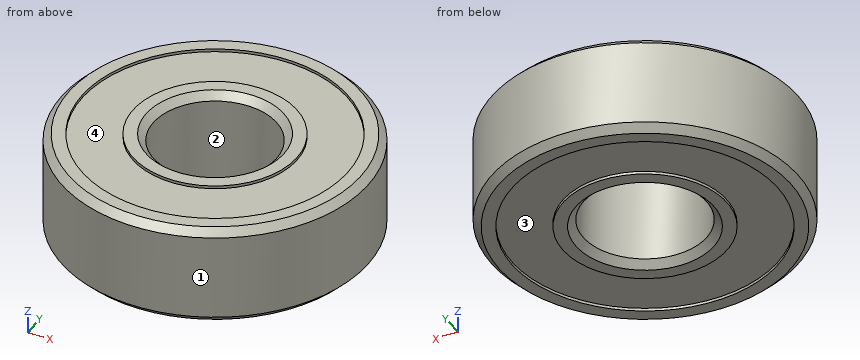
from build123d import *

# Parameters (mm, degrees)
ESQUISSE1_R        = 10.55
ESQUISSE1_R_2      = 9.15
BOSS_EXTRU_1_DEPTH = 3.45
ESQUISSE1_3_R      = 5.65
ESQUISSE1_3_R_2    = 4.25
BOSS_EXTRU_2_DEPTH = 3.45
ESQUISSE1_4_R      = 9.15
ESQUISSE1_4_R_2    = 5.65
BOSS_EXTRU_3_DEPTH = 3.25
CHANFREIN1_SIZE    = 0.5


with BuildPart() as part:
    # Esquisse1 → Boss.-Extru.1 (new body, symmetric)
    with BuildSketch(Plane.XY):
        Circle(ESQUISSE1_R)
        Circle(ESQUISSE1_R_2, mode=Mode.SUBTRACT)
    extrude(amount=BOSS_EXTRU_1_DEPTH, both=True)



with BuildPart() as body_2:
    # Esquisse1<3> → Boss.-Extru.2 (new body, symmetric)
    with BuildSketch(Plane.XY):
        Circle(ESQUISSE1_3_R)
        Circle(ESQUISSE1_3_R_2, mode=Mode.SUBTRACT)
    extrude(amount=BOSS_EXTRU_2_DEPTH, both=True)


with BuildPart() as part_1:
    add(part.part)

    add(body_2.part)  # Boss.-Extru.3 merges body 2
    # Esquisse1<4> → Boss.-Extru.3 (add, symmetric)
    with BuildSketch(Plane.XY):
        Circle(ESQUISSE1_4_R)
        Circle(ESQUISSE1_4_R_2, mode=Mode.SUBTRACT)
    extrude(amount=BOSS_EXTRU_3_DEPTH, both=True)

    # Chanfrein1
    chanfrein1_edges = [part_1.edges().sort_by_distance(p)[0] for p in [
        (-4.25, 0, -3.45),
        (-4.25, 0, 3.45),
        (-10.55, 0, -3.45),
        (-10.55, 0, 3.45),
    ]]
    chamfer(chanfrein1_edges, length=CHANFREIN1_SIZE)


solid = part_1.part
Verification items for the finished model (mm, model axes). Face numbers are marked on the shaded views. A direction names the side the tool comes from. Round coordinates to 2 decimals unless told otherwise and drop trailing zeros. Order: outer loops, then holes, each group sorted by start corner. A loop starts at its lowest first (then second) coordinate and runs counter-clockwise, first axis right, second up. Notation, with made-up numbers: (84, 82) -> (101, 82) arc R7 ccw to (101, 94) -> close; hole circle Ø8 at (11.25, -17.5). An arc over 180 degrees is marked (long way). Put each result on its own line as item: value.
1) Section check C-C (z = -1.5). Record the cut outline in (x, y), then the cut area to 3 significant figures.
Final values:
outline: circle Ø21.1 at (0, 0); hole circle Ø8.5 at (0, 0)
area: 293 mm^2
2) Mould release check, pull along X, two halves, no side actions. Record for the marked faces 1 and 2: +X half, -X half, draft (parallel to the pull), parting line (faces both ways), or undercut.
Final values:
face 1: parting line
face 2: undercut
3) Depth check by flat-ended pin: pin 1 (1.5 mm diameter, centred on y = 7, z = 1, fed in from -X); pin 2 (3 mm diameter, centred on x = 4.5, z = 0.5, fed in from +Y); pin 3 (1 mm diameter, centred on x = 8.5, z = 0.5, fed in from +Y). Enter the tip coordinate at first touch or a pass-through.
Final values:
pin 1: stops at x = -8.5
pin 2: stops at y = 10.11
pin 3: stops at y = 6.88
4) Set-up check for the marked faces 3 and 4: record each of +Z, -Z, +X, -X, +Y, -Y from which the full face is reachable in a straight line by a thin tool's end or side.
Final values:
face 3: -Z
face 4: +Z
5) Material ranges on line 1 (Y direction, x = 0, z = 3.3); line 2 (Y direction, x = 0, z = -3.4); line 3 (Y direction, x = 0, z = -0.8), recorded low to high.
Final values:
line 1: y = -10.2 to -9.15, -5.65 to -4.6, 4.6 to 5.65, 9.15 to 10.2
line 2: y = -10.1 to -9.15, -5.65 to -4.7, 4.7 to 5.65, 9.15 to 10.1
line 3: y = -10.55 to -4.25, 4.25 to 10.55
